```python
from build123d import *

# Parameters (mm, degrees)
F1_DEPTH = 10
F3_DEPTH = 25
F4_R     = 27.495097568
F5_DEPTH = 3
F6_R     = 1


# Not quite as in the source:
# - a feature names something its author has since deleted; it is built from what else it names


with BuildPart() as f1:
    # F0 (on Front) → F1 (new body)
    with BuildSketch(Plane.XZ):
        Polygon((11, 12.5), (8, 12.5), (8, -12.5), (-8, -12.5), (-8, 12.5), (-11, 12.5), (-11, -15.5), (11, -15.5), align=None)
        Polygon((25, -72.5), (11, -15.5), (-11, -15.5), (-25, -72.5), align=None)
    extrude(amount=F1_DEPTH)

    # F2 (on face) → F3 (cut)
    with BuildSketch(Plane.XZ.offset(10)):
        Polygon((-1.5, -15.5), (-7.9108356651, -15.5), (-21.9108356651, -72.5), (-1.5, -72.5), align=None)
        Polygon((1.5, -15.5), (1.5, -72.5), (21.9108356651, -72.5), (7.9108356651, -15.5), align=None)
    extrude(amount=-F3_DEPTH, mode=Mode.SUBTRACT)

    # F4 (on face) → F5 (join)
    with BuildSketch(Plane(origin=(0, 0, -72.5), x_dir=(1, 0, 0), z_dir=(0, 0, -1))):
        with Locations((0, 5)):
            Circle(F4_R)
    extrude(amount=F5_DEPTH)

    # F6
    f6_edges = [f1.edges().sort_by_distance(p)[0] for p in [
        (-8, -5, 12.5),
        (8, -5, 12.5),
        (11, -5, 12.5),
        (-11, -5, 12.5),
        (9.5, -10, 12.5),
        (-9.5, -10, 12.5),
        (9.5, 0, 12.5),
        (-9.5, 0, 12.5),
        (-11, 0, -1.5),
        (11, 0, -1.5),
        (11, -10, -1.5),
        (-11, -10, -1.5),
        (-18, -10, -44),
        (18, -10, -44),
        (-18, 0, -44),
        (18, 0, -44),
        (0, -10, -72.5),
        (23.455418, -10, -72.5),
        (14.910836, -10, -44),
        (4.705418, -10, -15.5),
        (1.5, -10, -44),
        (-1.5, -10, -44),
        (-4.705418, -10, -15.5),
        (-14.910836, -10, -44),
        (-23.455418, -10, -72.5),
        (-8, -10, 0),
        (0, -10, -12.5),
        (8, -10, 0),
        (23.455418, 0, -72.5),
        (14.910836, 0, -44),
        (4.705418, 0, -15.5),
        (1.5, 0, -44),
        (0, 0, -72.5),
        (-1.5, 0, -44),
        (-4.705418, 0, -15.5),
        (-14.910836, 0, -44),
        (-23.455418, 0, -72.5),
        (-8, 0, 0),
        (0, 0, -12.5),
        (8, 0, 0),
        (-27.495098, -5, -72.5),
        (-21.910836, -5, -72.5),
        (-25, -5, -72.5),
        (1.5, -5, -72.5),
        (-1.5, -5, -72.5),
        (25, -5, -72.5),
        (21.910836, -5, -72.5),
    ]]
    fillet(f6_edges, radius=F6_R)


solid = f1.part
```
Model file for the job. Use its own axes, mm. A direction names the side the tool comes from. Give positions to 0.01 mm unless a question says otherwise; leave off trailing zeros. Write each question's results on one line, items separated by ' | '.
(1) Probe line 1 along X through (y, z) = (-6, -22.5); line 2 along Z through (x, y) = (7, -18); line 3 along Y through (x, z) = (9.5, -9.5). List the from-to ranges inside material, lowest first.
Geometry results:
line 1: x = -12.72 to -9.63, -1.5 to 1.5, 9.63 to 12.72 | line 2: z = -75.5 to -72.5 | line 3: y = -10 to 0
(2) Flat gauge pins, fed straight in: pin 1 Ø9 at (y, z) = (-6, -4) entering from +X; pin 2 Ø14 at (x, z) = (-7, -39) entering from +Y; pin 3 Ø10 at (x, y) = (-3, 17) entering from +Z. Where does each tip first touch, or does it go through?
Geometry results:
pin 1: stops at x = 11 | pin 2: stops at y = 0 | pin 3: stops at z = -72.5
(3) Cut at A-A on y = -5. Give the number of separate pieces and of enclosed holes in the cut face, and give its area (3 significant figures).
Geometry results:
separate pieces: 1 | enclosed holes: 2 | area: 904 mm²
(4) Tool access for faces 1 (the flat face through (-8, -5, -1)), 2 (the flat face through (0, 0, -36)), 3 (the cylindrical face through (-15.1, -9.7, -43.57)): list every direction of +Z, -Z, +X, -X, +Y, -Y with a clear straight run to the whole face (end or side of a thin tool).
Geometry results:
face 1: +Z, +Y, -Y | face 2: +Z, +X, -X, +Y | face 3: -Y
(5) Pull direction X, two halves, no side cores. Call faces 4 (the flat face through (18, -5, -44)), 5 (the flat face through (1.5, -5, -43)), 6 (the cylindrical face through (14.918, -0.285, -42.768)), 7 (the flat face through (0, -10, -36)): released by +X, released by -X, zero draft, split by the parting line, or undercut.
Geometry results:
face 4: released by +X | face 5: undercut | face 6: undercut | face 7: zero draft
